Build history of the part. All positions in model axes, mm. A direction names the side the tool comes from. Give positions to 0.01 mm unless a question says otherwise; leave off trailing zeros. Order: outer loops, then holes, each group sorted by start corner. A loop starts at its lowest first (then second) coordinate and runs counter-clockwise, first axis right, second up. Notation, with made-up numbers: (85, -9) -> (101, -9) arc R15 ccw to (101, 16) -> close; hole circle Ø9 at (17.25, 42). An arc over 180 degrees is marked (long way). One line per question, with ' | ' between items. Start each with the question number.
(1) Cut at B-B (y = 47.5). Give the cut face in (x, z), then the cut area to 3 significant figures.
(2) Pin check, flat tips, straight feed: pin 1 Ø3 at (x, z) = (4, 5.5) entering from -Y; pin 2 Ø5 at (x, y) = (5, 4) entering from +Z. Stop position of each tip, or through.
(3) Pull direction Y, two halves, no side cores. Call faces 5 (the face through (5, 10, 5)), 6 (the face through (5, 75, 150)), 7 (the face through (5, 20, 5)): +Y half, -Y half, draft (parallel to the pull), parting line (faces both ways), or undercut.
(4) Which spindle directions (+Z, -Z, +X, -X, +Y, -Y) get a long thin tool onto all of the face, cutting with end or side? Do faces 1 (the face through (5, 55, 0)), 2 (the face through (5, 65, 10)), 3 (the face through (5, 5, 140)), 4 (the face through (5, 70, 145)). Say none if no direction does.
(5) Drill centre lines: L1, parallel to Y at x = 4.25, z = 144.5; L2, parallel to Z at x = 6.5, y = 3. Where is each one in solid material? Low to high. Write a range as from..to.
from build123d import *

# Parameters (mm, degrees)
ESQUISSE1_W                = 150
ESQUISSE1_H                = 80
BOSS_EXTRU_1_DEPTH         = 10
ESQUISSE2_W                = 10
ESQUISSE2_H                = 10
ENL_V_MAT_EXTRU_1_DEPTH    = 10
R_P_TITION_LIN_AIRE1_COUNT = 4
R_P_TITION_LIN_AIRE1_PITCH = 20


with BuildPart() as part:
    # Esquisse1 → Boss.-Extru.1 (new body)
    with BuildSketch(Plane(origin=(0, 0, 0), x_dir=(0, 0, -1), z_dir=(1, 0, 0))):
        with Locations((-75, 40)):
            Rectangle(ESQUISSE1_W, ESQUISSE1_H)
    extrude(amount=BOSS_EXTRU_1_DEPTH)

    # Esquisse2 → Enlèv. mat.-Extru.1 (cut)
    with BuildSketch(Plane.ZY):
        with Locations((5, 65)):
            Rectangle(ESQUISSE2_W, ESQUISSE2_H)
        with Locations((145, 65)):
            Rectangle(ESQUISSE2_W, ESQUISSE2_H)
    enl_v_mat_extru_1 = extrude(amount=-ENL_V_MAT_EXTRU_1_DEPTH, mode=Mode.SUBTRACT)

    # Répétition linéaire1: Enlèv. mat.-Extru.1 ×4
    with Locations(*[(0, -i * R_P_TITION_LIN_AIRE1_PITCH, 0) for i in range(1, R_P_TITION_LIN_AIRE1_COUNT)]):
        add(enl_v_mat_extru_1, mode=Mode.SUBTRACT)


solid = part.part
Result set:
1) outline: (0, 10) -> (10, 10) -> (10, 140) -> (0, 140) -> close | area: 1,300 mm2
2) pin 1: stops at y = 10 | pin 2: stops at z = 140
3) face 5: -Y half | face 6: draft | face 7: undercut
4) face 1: -Z, +X, -X, +Y, -Y | face 2: -Z, +X, -X | face 3: +Z, +X, -X, -Y | face 4: +Z, +X, -X
5) L1: y = 10..20, 30..40, 50..60, 70..80 | L2: z = 10..140
